Input: part model. Units: mm. Frame: model coordinates. Face numbers are marked on the shaded views. A direction names the side the tool comes from. Coordinates: 2 decimals unless noted, no trailing zeros. Write each loop counter-clockwise with the first axis right and the second up, starting at its lowest first coordinate (ties: lowest second). Pieces come first, ordered by that corner, then holes. Notation, with made-up numbers: (28.5, -35.75) -> (34.5, -35.75) arc R24 cw to (34.5, 2.25) -> close; hole circle Ø5 at (-17.75, -38.75). An arc over 180 degrees is marked (long way). Use one line per item in the form item = value. Start each with the question number.
(1) Pull-direction query (X, two-part tool) for the marked faces 3 and 4; classes: released by +X, released by -X, zero draft, split by the parting line, or undercut.
(2) Ray query, line 1 along Z through (x, y) = (-119.5, 33.5); line 2 along X through (y, z) = (132, -1); line 3 along Z through (x, y) = (27.5, -71). Return the intervals inside material, ascending.
(3) Cut plane C-C on x = -60.5. Return the cut outline in (y, z).
(4) First-contact query: pin 1 (1.5 mm diameter, centred on y = 178, z = -1, fed in from +X) (3 decimals); pin 2 (3.5 mm diameter, centred on y = 142, z = -1.5, fed in from +X); pin 3 (3.5 mm diameter, centred on y = 135.5, z = -1.5, fed in from -X); pin 4 (4 mm diameter, centred on x = -116.5, z = 2.5, fed in from +Y). Flat tips, straight axial feed; report the tip coordinate or a pass-through.
(5) Cut plane A-A on x = 0. Return the cut outline in (y, z), plus the area to 3 significant figures.
(6) Cut plane B-B on y = 124. Return the cut outline in (x, z).
(7) Set-up query: the marked faces 1 and 2. Return all of +Z, -Z, +X, -X, +Y, -Y with unobstructed straight access to the full face (end or side cutting, diameter ignored); none if empty.
(8) Cut plane D-D on x = 123. Return the cut outline in (y, z).
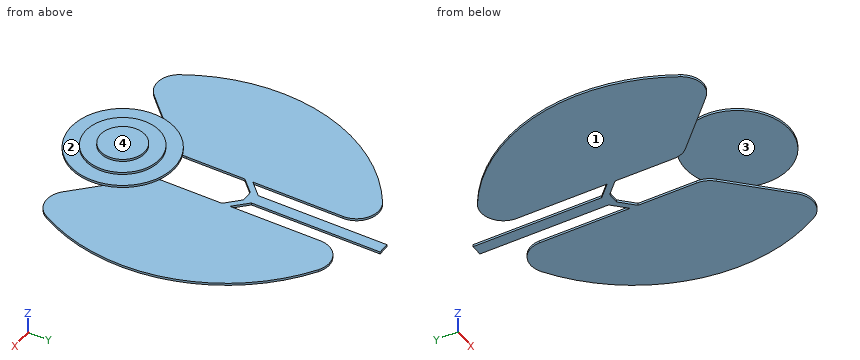
```python
from build123d import *

# Parameters (mm, degrees)
BOSS_EXTRUDE2_DEPTH = 3
SKETCH4_R           = 70
BOSS_EXTRUDE3_DEPTH = 3
SKETCH5_R           = 50
BOSS_EXTRUDE4_DEPTH = 3
SKETCH6_R           = 30
BOSS_EXTRUDE5_DEPTH = 3


with BuildPart() as part:
    # Sketch3 → Boss-Extrude2 (new body)
    with BuildSketch(Plane.XY):
        with BuildLine():
            Line((-7.732951968, 171.945409862), (-7.732951968, 79.732573414))
            Line((-7.732951968, 79.732573414), (-25.727277728, 61.647728335))
            Line((-25.727277728, 61.647728335), (-25.727277728, 183.232578721))
            ThreePointArc((-25.727277728, 183.232578721), (-41.33367569, 209.554133014), (-71.915559085, 208.490043889))
            ThreePointArc((-71.915559085, 208.490043889), (-174.808712355, 64.246349724), (-149.59307925, -111.131574039))
            ThreePointArc((-149.59307925, -111.131574039), (-127.490841861, -125.869970667), (-102.352099339, -117.280857953))
            Line((-102.352099339, -117.280857953), (-34.460919249, -49.048155569))
            ThreePointArc((-34.460919249, -49.048155569), (-27.996511832, -39.333965794), (-25.727277728, -27.888240705))
            Line((-25.727277728, -27.888240705), (-25.727277728, 50.916062024))
            Line((-25.727277728, 50.916062024), (-7.732951969, 69.000907103))
            Line((-7.732951969, 69.000907103), (7.732951969, 69.000907103))
            Line((7.732951969, 69.000907103), (25.727277728, 50.916062024))
            Line((25.727277728, 50.916062024), (25.727277728, -27.888240705))
            ThreePointArc((25.727277728, -27.888240705), (27.996511832, -39.333965794), (34.460919249, -49.048155569))
            Line((34.460919249, -49.048155569), (102.352099339, -117.280857953))
            ThreePointArc((102.352099339, -117.280857953), (127.490841861, -125.869970667), (149.59307925, -111.131574039))
            ThreePointArc((149.59307925, -111.131574039), (174.808712355, 64.246349724), (71.915559085, 208.490043889))
            ThreePointArc((71.915559085, 208.490043889), (41.33367569, 209.554133014), (25.727277728, 183.232578721))
            Line((25.727277728, 183.232578721), (25.727277728, 61.647728335))
            Line((25.727277728, 61.647728335), (7.732951968, 79.732573414))
            Line((7.732951968, 79.732573414), (7.732951968, 171.945409862))
            Line((7.732951968, 171.945409862), (7.732951968, 252.911456322))
            Line((7.732951968, 252.911456322), (-7.732951968, 252.911456322))
            Line((-7.732951968, 252.911456322), (-7.732951968, 171.945409862))
        make_face()
    extrude(amount=-BOSS_EXTRUDE2_DEPTH)

    # Sketch4 → Boss-Extrude3 (add)
    with BuildSketch(Plane.XY):
        with Locations(Location((0, -98.03156951, 0), (0, 0, 167.733969659))):
            Circle(SKETCH4_R)
    extrude(amount=BOSS_EXTRUDE3_DEPTH)

    # Sketch5 → Boss-Extrude4 (add)
    with BuildSketch(Plane.XY.offset(3)):
        with Locations((0, -98.03156951)):
            Circle(SKETCH5_R)
    extrude(amount=BOSS_EXTRUDE4_DEPTH)

    # Sketch6 → Boss-Extrude5 (add)
    with BuildSketch(Plane.XY.offset(6)):
        with Locations((0, -98.03156951)):
            Circle(SKETCH6_R)
    extrude(amount=BOSS_EXTRUDE5_DEPTH)


solid = part.part
```
Values:
q1.face_3 = undercut
q1.face_4 = zero draft
q2.line_1 = -3 to 0
q2.line_2 = -146.72 to -25.73, -7.73 to 7.73, 25.73 to 146.72
q2.line_3 = 0 to 6
q3.outline = (-133.24, 0) -> (-75.22, 0) -> (-75.22, -3) -> (212.85, -3) -> (212.85, 0) -> (-62.82, 0) -> (-62.82, 3) -> (-133.24, 3) -> close
q4.pin_1 = 110.935
q4.pin_2 = 141.45
q4.pin_3 = -145.64
q4.pin_4 = through
q5.outline = (-168.03, 0) -> (-28.03, 0) -> (-28.03, 3) -> (-48.03, 3) -> (-48.03, 6) -> (-68.03, 6) -> (-68.03, 9) -> (-128.03, 9) -> (-128.03, 6) -> (-148.03, 6) -> (-148.03, 3) -> (-168.03, 3) -> close; (69, -3) -> (252.91, -3) -> (252.91, 0) -> (69, 0) -> close
q5.area = 1,450 mm2
q6.outline = (-151.39, -3) -> (-25.73, -3) -> (-25.73, 0) -> (-151.39, 0) -> close; (-7.73, -3) -> (7.73, -3) -> (7.73, 0) -> (-7.73, 0) -> close; (25.73, -3) -> (151.39, -3) -> (151.39, 0) -> (25.73, 0) -> close
q7.face_1 = -Z, +X, -X, +Y, -Y
q7.face_2 = +Z
q8.outline = (-126.11, -3) -> (164.39, -3) -> (164.39, 0) -> (-126.11, 0) -> close
